```python
from build123d import *

# Parameters (mm, degrees)
FILLET1_R = 0.1


with BuildPart() as part:
    # Sketch1 → Revolve1 (revolve)
    with BuildSketch(Plane.XY):
        with BuildLine():
            Line((0, 0), (10, 0))
            Line((10, 0), (10, 2.325))
            ThreePointArc((10, 2.325), (9.831586399, 2.731586399), (9.425, 2.9))
            ThreePointArc((9.425, 2.9), (9.354289322, 2.870710678), (9.325, 2.8))
            Line((9.325, 2.8), (8.85, 2.8))
            Line((8.85, 2.8), (8.85, 3.1))
            ThreePointArc((8.85, 3.1), (8.820710678, 3.170710678), (8.75, 3.2))
            Line((8.75, 3.2), (0, 3.2))
            Line((0, 3.2), (0, 0))
        make_face()
    revolve(axis=Axis((0, 0, 0), (0, 1, 0)))

    # Fillet1
    fillet1_edges = [part.edges().sort_by_distance(p)[0] for p in [
        (-10, 0, 0),
    ]]
    fillet(fillet1_edges, radius=FILLET1_R)


solid = part.part
```
The listing builds one solid part. Answer for the finished solid, in the listing's coordinates (mm). Coordinates: 2 decimals unless noted, no trailing zeros. Loops run counter-clockwise (first coordinate to the right, second up) from the corner with the lowest first, then second, coordinate; pieces in that order, holes last. Notation, with made-up numbers: (-18, 17.5) -> (35, 17.5) arc R9 cw to (35, 31.5) -> close; hole circle Ø9 at (-26.75, 57.5). An arc over 180 degrees is marked (long way). Return JSON: item names as keys, results as strings. Group by question number.
(1) Determine the mould class of faces 1 (the flat face through (0, 0, 0)), 2 (the cylindrical face through (8.44, 2.95, -2.66)), 3 (the cylindrical face through (-2.17, 1.23, 9.76)) for opening direction X: released by +X, released by -X, zero draft, split by the parting line, or undercut.
(2) A cutting plane is placed at A-A on y = 0.9. Write down the section's boundary in (x, z), and give its area (3 significant figures).
(3) Find the intervals of material crossed by probe 1 along Z at (x, y) = (0, 0.45); probe 2 along Y at (x, z) = (-2.25, -8.5); probe 3 along X at (y, z) = (1.5, 1), in increasing order. Write a range as from..to.
(4) Given pin 1 Ø5 at (x, z) = (7.5, -3.5) entering from -Y; pin 2 Ø1 at (x, y) = (-1.5, 1.5) entering from +Z, each flat-ended and moving along its own axis, determine where each tip first touches the part or whether it passes through.
The answers:
{
 "1": {"face 1": "zero draft", "face 2": "undercut", "face 3": "split by the parting line"},
 "2": {"outline": "circle Ø20 at (0, 0)", "area": "314 mm^2"},
 "3": {"probe 1": "z = -10..10", "probe 2": "y = 0..3.19", "probe 3": "x = -9.95..9.95"},
 "4": {"pin 1": "stops at y = 0", "pin 2": "stops at z = 9.95"}
}
